Autodesk Inventor part; units mm, degrees
ref_plane "Work Plane1" through (0, 0, 16) normal (0, 0, 1) x (1, 0, 0)
ref_plane "YZ Plane" through (0, 0, 0) normal (1, 0, 0) x (0, 1, 0)
ref_plane "XZ Plane" through (0, 0, 0) normal (0, 1, 0) x (-1, 0, 0)
sketch "Sketch1" plane through (0, 0, 0) normal (0, 0, 1) x (1, 0, 0)
  line L0 (-36.8533, 0) -> (46.8153, 0) construction
  line L1 (0, -29.8808) -> (0, 4.9801) construction
  line L2 (0, 0) -> (24.6516, -24.6516) construction
  line L3 (0, 0) -> (34.8626, 0) construction
  line L4 (0, -24.9006) -> (16.8, -24.9006)
  line L5 (16.8, -24.9006) -> (16.8, -21.2406)
  line L6 (16.8, -21.2406) -> (19.0203, -19.0203)
  line L7 (24.9006, 0) -> (24.9006, -16.8)
  line L8 (24.9006, -16.8) -> (21.2406, -16.8)
  line L9 (21.2406, -16.8) -> (19.0203, -19.0203)
  line L10 (0, 0) -> (-24.6516, -24.6516) construction
  line L11 (0, -24.9006) -> (-16.8, -24.9006)
  line L12 (-16.8, -24.9006) -> (-16.8, -21.2406)
  line L13 (-16.8, -21.2406) -> (-19.0203, -19.0203)
  line L14 (-24.9006, 0) -> (-24.9006, -16.8)
  line L15 (-24.9006, -16.8) -> (-21.2406, -16.8)
  line L16 (-21.2406, -16.8) -> (-19.0203, -19.0203)
  arc A0 (-14, 0) -> (14, 0) centre (0, 0) ccw
  line L17 (0, 0) -> (14, 0) construction
  line L18 (0, 0) -> (-14, 0) construction
  line L19 (-14, 0) -> (-24.9006, 0)
  line L20 (14, 0) -> (24.9006, 0)
  dimension "d0" = 45
  dimension "d1" = 16.8
  dimension "d2" = 3.66
  dimension "d4" = 3.14
  dimension "d5" = 14
  dimension "d6" = 180
extrude "Extrusion1" add sketch "Sketch1" along normal blind 5
sketch "Sketch3" plane through (-24.9006, 0, 0) normal (0, 1, 0) x (1, 0, 0)
  line L0 (10.9006, 0) -> (0, 0) construction
  line L1 (0, 0) -> (0, -5) construction
  line L2 (10.9006, -5) -> (0, -5) construction
  line L3 (10.9006, 0) -> (10.9006, -5) construction
  line L4 (38.9006, 0) -> (10.9006, 0) construction
  line L5 (10.9006, 0) -> (10.9006, -5) construction
  line L6 (38.9006, -5) -> (10.9006, -5) construction
  line L7 (38.9006, 0) -> (38.9006, -5) construction
  line L8 (49.8013, 0) -> (38.9006, 0) construction
  line L9 (38.9006, 0) -> (38.9006, -5) construction
  line L10 (49.8013, -5) -> (38.9006, -5) construction
  line L11 (49.8013, 0) -> (49.8013, -5) construction
  line L12 (24.9006, 18.5006) -> (24.9006, -23.5037) construction
  arc A0 (10.9006, 0) -> (24.9006, -14) centre (24.9006, 0) ccw
  arc A1 (8.9006, 0) -> (24.9006, -16) centre (24.9006, 0) ccw
  line L13 (24.9006, -16) -> (24.9006, -14)
  line L14 (10.9006, 0) -> (0, 0)
  line L15 (8.9006, 0) -> (10.9006, 0)
  dimension "d11" = 2
revolve "Revolution2" add sketch "Sketch3" angle 180 about axis through (0, 0, -10) along (0, 0, 1)
ref_plane "Work Plane1" through (0, 0, 16) normal (0, 0, 1) x (1, 0, 0)
sketch "Sketch5" plane through (24.9006, 0, 5) normal (0, 1, 0) x (1, 0, 0)
  line L0 (0, 0) -> (-9.7019, 0) construction
  line L1 (0, 5) -> (0, 0) construction
  line L2 (0, 5) -> (-10.9006, 5) construction
  arc A0 (-38.9006, 5) -> (-10.9006, 5) centre (-24.9006, 5) ccw construction
  line L3 (-38.9006, 5) -> (-49.8013, 5) construction
  line L4 (-49.8013, 5) -> (-49.8013, 0) construction
  line L5 (-40.0993, 0) -> (-49.8013, 0) construction
  arc A1 (-40.0993, 0) -> (-9.7019, 0) centre (-24.9006, 5) ccw construction
  arc A2 (-38.9006, 5) -> (-10.9006, 5) centre (-24.9006, 5) ccw construction
  line L6 (-10.9006, 5) -> (-38.9006, 5) construction
  line L7 (-24.9006, 25) -> (-24.9006, -17) construction
  line L8 (-24.9006, -6) -> (-35.7006, -6)
  line L9 (-35.7006, -6) -> (-35.7006, -8.1)
  line L10 (-35.7006, -8.1) -> (-24.9006, -8.1)
  line L11 (-24.9006, -8.1) -> (-24.9006, -6)
  arc A3 (-10.9006, 5) -> (-38.9006, 5) centre (-24.9006, 5) ccw construction
  line L12 (-24.9006, 19) -> (-24.9006, -6) construction
  line L13 (-24.9006, 19) -> (0.0994, 19) construction
  line L14 (-34.7006, -6) -> (-33.5609, -6)
  line L15 (-33.5609, -6) -> (-33.5609, -4.998)
  line L16 (-33.5609, -4.998) -> (-34.7006, -4.998)
  line L17 (-34.7006, -4.998) -> (-34.7006, -6)
  arc A4 (-38.9006, 5) -> (-10.9006, 5) centre (-24.9006, 5) ccw
  line L18 (-24.9006, -8.1) -> (-34.087, -8.1)
  line L19 (-34.087, -8.1) -> (-34.087, -11)
  line L20 (-34.087, -11) -> (-24.9006, -11)
  line L21 (-24.9006, -11) -> (-24.9006, -8.1)
  arc A5 (-40.0993, 0) -> (-9.7019, 0) centre (-24.9006, 5) ccw
  dimension "d16" = 10.8
  dimension "d17" = 2.1
  dimension "d19" = 25
  dimension "d20" = 90
  dimension "d21" = 1
revolve "Revolution3" cut sketch "Sketch5" angle 360 about axis through (0, 0, -10) along (0, 0, 1) contours L11 L10 A4 L8 | A4 L10 A5 L9 L8 | L8 L17 A4 | L21 A4 L10 | A4 L21 A5 L10 | L10 L9 A5
sketch "Sketch6" plane through (-24.9006, 0, 5) normal (0, 1, 0) x (1, 0, 0)
  line L0 (14.1006, -6.8051) -> (14.1006, -6) construction
  line L1 (14.1006, -6) -> (15.1006, -6) construction
  line L2 (15.1006, -6) -> (15.1006, -4.998) construction
  arc A0 (10.9006, 5) -> (15.1006, -4.998) centre (24.9006, 5) ccw construction
  line L3 (10.9006, 5) -> (0, 5) construction
  line L4 (0, 5) -> (0, 0) construction
  line L5 (9.7019, 0) -> (0, 0) construction
  arc A1 (9.7019, 0) -> (14.1006, -6.8051) centre (24.9006, 5) ccw construction
  line L6 (24.9006, 7.4176) -> (24.9006, -9.5058) construction
  arc A2 (9.7019, 0) -> (14.1006, -6.8051) centre (24.9006, 5) ccw
  line L7 (13.2817, -6) -> (13.2817, -9.314)
  line L8 (14.1006, -6) -> (24.9006, -6) construction
  line L9 (24.9006, -6) -> (24.9006, -8) construction
  line L10 (24.9006, -8) -> (14.1006, -8) construction
  line L11 (14.1006, -8) -> (14.1006, -6) construction
  line L12 (35.7006, -6) -> (14.1006, -6) construction
  line L13 (14.1006, -6) -> (24.9006, -6) construction
  line L14 (24.9006, -6) -> (24.9006, -11.2) construction
  line L15 (24.9006, -11.2) -> (14.1006, -11.2) construction
  line L16 (14.1006, -11.2) -> (14.1006, -6) construction
  arc A3 (14.1006, -8) -> (24.9006, -11.2) centre (24.9006, 8.625) ccw construction
  line L17 (14.1006, -6.8051) -> (14.1006, -8)
  line L18 (13.2817, -9.314) -> (15.1006, -9.314)
  line L19 (15.1006, -9.314) -> (15.1006, -8.6084)
  line L20 (15.1006, -8.6084) -> (14.1006, -8)
  line L21 (13.2817, -6) -> (14.1006, -6)
  line L22 (35.7006, -6.8051) -> (14.1006, -6.8051)
  line L23 (14.1006, -6.8051) -> (14.1006, -6)
  dimension "d23" = 2
  dimension "d24" = 5.2
revolve "Revolution4" add sketch "Sketch6" angle 180 about axis through (0, 0, -10) along (0, 0, 1) contours A2 L17 L20 L19 L18 L7
sketch "Sketch7" plane through (0, 0, 0) normal (0, 0, -1) x (-1, 0, 0)
  line L0 (-24.9006, 0) -> (-14, 0)
  line L1 (-24.9006, -16.8) -> (-24.9006, 0)
  line L2 (-21.2406, -16.8) -> (-24.9006, -16.8)
  line L3 (-16.8, -21.2406) -> (-21.2406, -16.8)
  line L4 (-16.8, -24.9006) -> (-16.8, -21.2406)
  line L5 (16.8, -24.9006) -> (-16.8, -24.9006)
  line L6 (16.8, -21.2406) -> (16.8, -24.9006)
  line L7 (21.2406, -16.8) -> (16.8, -21.2406)
  line L8 (24.9006, -16.8) -> (21.2406, -16.8)
  line L9 (24.9006, 0) -> (24.9006, -16.8)
  line L10 (14, 0) -> (24.9006, 0)
  arc A0 (-14, 0) -> (14, 0) centre (0, 0) ccw
extrude "Extrusion3" add sketch "Sketch7" along normal blind 7
sketch "Skizze8" plane through (0, 0, 5) normal (0, 0, 1) x (1, 0, 0)
  arc A0 (-15.1987, 0) -> (15.1987, 0) centre (0, 0) ccw construction
  line L0 (-15.1987, 0) -> (-24.9006, 0) construction
  line L1 (-24.9006, 0) -> (-24.9006, -16.8) construction
  line L2 (-24.9006, -16.8) -> (-21.2406, -16.8)
  line L3 (-21.2406, -16.8) -> (-16.8, -21.2406)
  line L4 (-16.8, -21.2406) -> (-16.8, -24.9006)
  line L5 (-16.8, -24.9006) -> (16.8, -24.9006) construction
  line L6 (16.8, -24.9006) -> (16.8, -21.2406)
  line L7 (16.8, -21.2406) -> (21.2406, -16.8)
  line L8 (21.2406, -16.8) -> (24.9006, -16.8)
  line L9 (24.9006, -16.8) -> (24.9006, 0) construction
  line L10 (24.9006, 0) -> (15.1987, 0) construction
  line L11 (25.0006, 0.1) -> (25.0006, -16.9) construction
  line L12 (25.0006, -16.9) -> (21.2821, -16.9)
  line L13 (21.2821, -16.9) -> (16.9, -21.2821)
  line L14 (16.9, -21.2821) -> (16.9, -25.0006)
  line L15 (16.9, -25.0006) -> (-16.9, -25.0006) construction
  line L16 (-16.9, -25.0006) -> (-16.9, -21.2821)
  line L17 (-16.9, -21.2821) -> (-21.2821, -16.9)
  line L18 (-21.2821, -16.9) -> (-25.0006, -16.9)
  line L19 (-25.0006, -16.9) -> (-25.0006, 0.1) construction
  line L20 (-25.0006, 0.1) -> (-15.0984, 0.1) construction
  arc A1 (-15.0984, 0.1) -> (15.0984, 0.1) centre (0, 0) ccw construction
  line L21 (15.0984, 0.1) -> (25.0006, 0.1) construction
  line L22 (-24.9006, -16.8) -> (-24.9006, -16.9)
  line L23 (-16.8, -24.9006) -> (-16.9, -24.9006)
  line L24 (16.8, -24.9006) -> (-16.8, -24.9006)
  line L25 (16.8, -24.9006) -> (16.9, -24.9006)
  line L26 (24.9006, 0) -> (24.9006, -16.8)
  line L27 (24.9006, -16.8) -> (24.9006, -16.9)
  point P0 (0, 0)
  dimension "d0" = 45
  dimension "d1" = 16.8
  dimension "d2" = 3.66
  dimension "d4" = 3.14
  dimension "d5" = 14
  dimension "d6" = 180
  dimension "d28" = 0.1
extrude "IM_offset" add sketch "Skizze8" against normal up to surface (12 mm away)
properties part number "20_Cube_Insert_Eye_Lens_v3"
Read the model definition and answer for the solid it produces. Units are mm, in the model's axes. A direction names the side the tool comes from. Round coordinates to 2 decimals unless told otherwise and drop trailing zeros. Write each loop counter-clockwise with the first axis right and the second up, starting at its lowest first coordinate (ties: lowest second). Pieces come first, ordered by that corner, then holes. Notation, with made-up numbers: (17, -25.5) -> (71, -25.5) arc R10 ccw to (71, -15.5) -> close; hole circle Ø5 at (81, 3.25). An arc over 180 degrees is marked (long way). Answer in a Markdown table with one row per item. Add a question column.
1) Consider line 1 (Z direction, x = 18.5, y = -15.5); line 2 (X direction, y = -7, z = -0.5); line 3 (Y direction, x = -22.5, z = 0.5). Determine where each line is inside the solid, lowest interval first.
2) Find section A-A, the plane z = -4.5. Determine the outline of the cut face in (x, y).
3) Given P1, Ø1, axis at x = 15.5, z = 8.5, coming from the +Y side; P2, Ø5, axis at y = -4.5, z = 12, coming from the -X side; P3, Ø1.1, axis at y = -22.5, z = 0.5, coming from the +X side; P4, Ø1.8, axis at x = -23.5, z = -3.5, coming from the -Y side, each flat-ended and moving along its own axis, determine where each tip first touches the part or whether it passes through.
4) Which of the six approach directions +Z, -Z, +X, -X, +Y, -Y give full straight-line access (tool end or side, diameter ignored) to faces 5 (the face through (23, -16.9, -1)), 6 (the face through (-23, -16.9, -1)), 7 (the face through (0, -14, -3)), 8 (the face through (0, -18, 5))?
5) Determine the mould class of faces 1 (the face through (0.219, -9.971, 13.503)), 2 (the face through (16.9, -23, -1)), 3 (the face through (0, -15, -7)), 4 (the face through (-0.2, -10.8, 12)) for opening direction Z: pulls with the +Z half, pulls with the -Z half, needs draft (parallel to the pull), parting line crosses it, or undercut.
6) Find section D-D, the plane y = -19.25. Determine the outline of the cut face in (x, z), and give its area (3 significant figures).
7) Find section B-B, the plane x = -13.5. Determine the outline of the cut face in (y, z), and give its area (3 significant figures).
8) Find section C-C, the plane z = 2. Determine the outline of the cut face in (x, y).
Findings below:
| question | item | result |
|---|---|---|
| 1 | line 1 | -7 to 5 |
| 1 | line 2 | -24.9 to -12.12, 12.12 to 24.9 |
| 1 | line 3 | -16.9 to 0 |
| 2 | outline | (-24.9, -16.9) -> (-21.28, -16.9) -> (-16.9, -21.28) -> (-16.9, -24.9) -> (16.9, -24.9) -> (16.9, -21.28) -> (21.28, -16.9) -> (24.9, -16.9) -> (24.9, 0) -> (14, 0) arc R14 cw to (-14, 0) -> (-24.9, 0) -> close |
| 3 | P1 | through |
| 3 | P2 | x = -12.23 |
| 3 | P3 | x = 16.9 |
| 3 | P4 | y = -16.9 |
| 4 | face 5 | +Z, -Z, +X, -Y |
| 4 | face 6 | +Z, -Z, -X, -Y |
| 4 | face 7 | -Z, +Y |
| 4 | face 8 | +Z, -Y |
| 5 | face 1 | undercut |
| 5 | face 2 | needs draft |
| 5 | face 3 | pulls with the -Z half |
| 5 | face 4 | undercut |
| 6 | outline | (-18.93, -7) -> (18.93, -7) -> (18.93, 5) -> (-18.93, 5) -> close |
| 6 | area | 454 mm² |
| 7 | outline | (-24.9, -7) -> (-3.71, -7) -> (-3.71, 0) arc R3.71 cw to (0, 3.71) -> (0, 8.59) arc R8.59 ccw to (-6.98, 5) -> (-24.9, 5) -> close |
| 7 | area | 280 mm² |
| 8 | outline | (-24.9, -16.9) -> (-21.28, -16.9) -> (-16.9, -21.28) -> (-16.9, -24.9) -> (16.9, -24.9) -> (16.9, -21.28) -> (21.28, -16.9) -> (24.9, -16.9) -> (24.9, 0) -> (13.86, 0) arc R13.86 cw to (-13.86, 0) -> (-24.9, 0) -> close |
